Can you work these out from the drawing? Everything is in mm from the part's minimum corner. A direction names the side the tool comes from. Coordinates: 2 decimals unless noted, no trailing zeros. Loops run counter-clockwise (first coordinate to the right, second up) from the corner with the lowest first, then second, coordinate; pieces in that order, holes last.
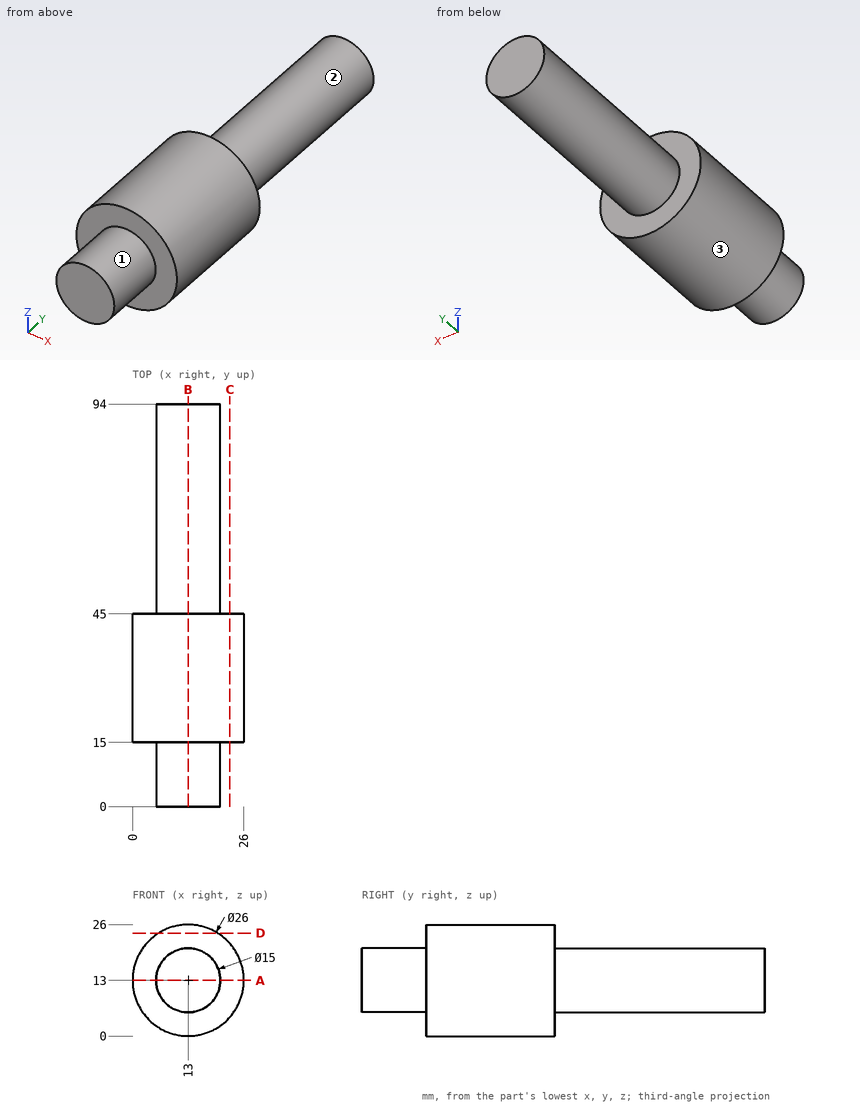
1. On a 3-axis mill with a long thin cutter (end or side, diameter ignored), from which of +Z, -Z, +X, -X, +Y, -Y can I reach the whole of each face in a straight line? I mean the marked faces 1, 2 and 3. Say none if no direction works.
2. I want a section at C-C (x = 22.75). Please give me the cut outline in (y, z), then the cut area to 3 significant figures.
3. I want a section at B-B (x = 13). Please give me the cut outline in (y, z), then the cut area to 3 significant figures.
4. I need wall thicknesses on line 1 along Y through (x, z) = (18, 4.25); line 2 along X through (y, z) = (41.5, 13.5). Which ranges of each line are inside material? Lowest first, please.
5. For pin 1 (10 mm diameter, centred on x = 16.5, z = 16, fed in from -Y); pin 2 (1 mm diameter, centred on y = 68, z = 13, fed in from -X); pin 3 (2 mm diameter, centred on x = 21.5, z = 8, fed in from -Y); pin 4 (3 mm diameter, centred on y = 81, z = 7, fed in from -X), each with a flat end and sliding along its axis, tell me the tip position at first contact or that it passes through.
6. I want a section at A-A (z = 13). Please give me the cut outline in (x, y), then the cut area to 3 significant figures.
7. I want a section at D-D (z = 24). Please give me the cut outline in (x, y), then the cut area to 3 significant figures.
Response values:
1. face 1: -Y
1. face 2: +Y
1. face 3: +Y, -Y
2. outline: (15, 4.4) - (45, 4.4) - (45, 21.6) - (15, 21.6) - close
2. area: 516 mm2
3. outline: (0, 5.5) - (15, 5.5) - (15, 0) - (45, 0) - (45, 5.5) - (94, 5.5) - (94, 20.5) - (45, 20.5) - (45, 26) - (15, 26) - (15, 20.5) - (0, 20.5) - close
3. area: 1,740 mm2
4. line 1: y = 15 to 45
4. line 2: x = 0.01 to 25.99
5. pin 1: stops at y = 0
5. pin 2: stops at x = 5.5
5. pin 3: stops at y = 15
5. pin 4: stops at x = 7
6. outline: (0, 15) - (5.5, 15) - (5.5, 0) - (20.5, 0) - (20.5, 15) - (26, 15) - (26, 45) - (20.5, 45) - (20.5, 94) - (5.5, 94) - (5.5, 45) - (0, 45) - close
6. area: 1,740 mm2
7. outline: (6.07, 15) - (19.93, 15) - (19.93, 45) - (6.07, 45) - close
7. area: 416 mm2
